from build123d import *

# Parameters (mm, degrees)
BOSS_EXTRUDE1_DEPTH         = 19.05
FILLET1_R                   = 6.35
F_29_0_136_DIAMETER_HOLE1_D = 3.4544


with BuildPart() as part:
    # Sketch1 → Boss-Extrude1 (new body)
    with BuildSketch(Plane.XY):
        with BuildLine():
            ThreePointArc((22.356689849, -6.35), (-23.241, 0), (22.356689849, 6.35))
            Line((22.356689849, 6.35), (57.15, 6.35))
            Line((57.15, 6.35), (57.15, 9.525))
            Line((57.15, 9.525), (24.638981939, 9.525))
            ThreePointArc((24.638981939, 9.525), (-26.416, 0), (24.638981939, -9.525))
            Line((24.638981939, -9.525), (57.15, -9.525))
            Line((57.15, -9.525), (57.15, -6.35))
            Line((57.15, -6.35), (22.356689849, -6.35))
        make_face()
    extrude(amount=BOSS_EXTRUDE1_DEPTH)

    # Fillet1
    fillet1_edges = [part.edges().sort_by_distance(p)[0] for p in [
        (22.356689849, 6.35, 9.525),
        (22.356689849, -6.35, 9.525),
        (24.638981939, -9.525, 9.525),
        (24.638981939, 9.525, 9.525),
    ]]
    fillet(fillet1_edges, radius=FILLET1_R)

    # #29 (0.136) Diameter Hole1 (through all)
    with Locations(Plane(origin=(0, 9.525, 0), x_dir=(1, 0, 0), z_dir=(0, 1, 0))):
        with Locations((33.655, -9.525), (52.705, -9.525)):
            Hole(F_29_0_136_DIAMETER_HOLE1_D / 2)


solid = part.part
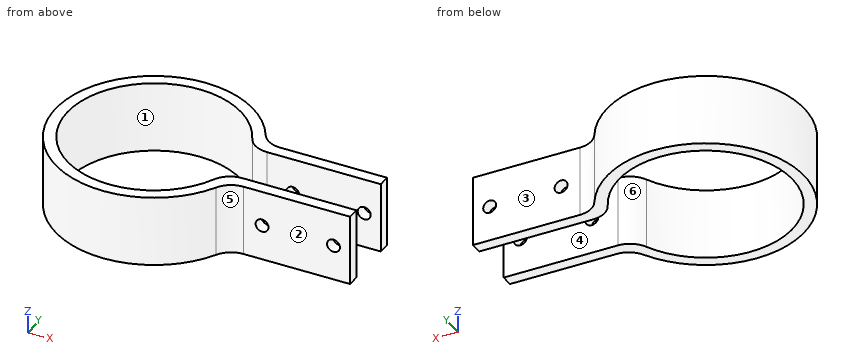
Verification items for the finished model (mm, model axes). Face numbers are marked on the shaded views. A direction names the side the tool comes from. Coordinates: 2 decimals unless noted, no trailing zeros. Loops run counter-clockwise (first coordinate to the right, second up) from the corner with the lowest first, then second, coordinate; pieces in that order, holes last. Notation, with made-up numbers: (-24, 35.5) -> (25, 35.5) arc R29 cw to (25, 62.5) -> close; hole circle Ø11 at (30, -2.75). An arc over 180 degrees is marked (long way). Answer as CSV lines item,"result".
1) Thickness scan on L1, parallel to Y at x = 0, z = 4; L2, parallel to Y at x = 34.5, z = 14.5 (3 decimals); L3, parallel to X at y = -7, z = 5.5. Record the ranges inside material, lowest first. Write a range as from..to.
Found:
L1,"y = -26.42..-23.24, 23.24..26.42"
L2,"y = -9.525..-6.35, 6.35..9.525"
L3,"x = -25.47..-22.16, 23.93..57.15"
2) Cross-section at A-A, the plane x = 0. Record the cut outline in (y, z).
Found:
outline,"(-26.42, 0) -> (-23.24, 0) -> (-23.24, 19.05) -> (-26.42, 19.05) -> close; (23.24, 0) -> (26.42, 0) -> (26.42, 19.05) -> (23.24, 19.05) -> close"
3) Release check for a two-part mould opening along Y. For the marked faces 1, 2 and 3 record: +Y half, -Y half, draft (parallel to the pull), parting line (faces both ways), or undercut.
Found:
face 1,"undercut"
face 2,"-Y half"
face 3,"+Y half"
4) Cross-section at B-B, the plane z = 2.75. Record the cut outline in (x, y) (3 decimals).
Found:
outline,"(20.992, -9.975) arc R23.241 cw (long way) to (20.992, 9.975) arc R6.35 ccw to (26.727, 6.35) -> (57.15, 6.35) -> (57.15, 9.525) -> (28.663, 9.525) arc R6.35 cw to (23.109, 12.798) arc R26.416 ccw (long way) to (23.109, -12.798) arc R6.35 cw to (28.663, -9.525) -> (57.15, -9.525) -> (57.15, -6.35) -> (26.727, -6.35) arc R6.35 ccw to start"
5) Depth check by flat-ended pin: pin 1 (5 mm diameter, centred on x = 18, z = 8, fed in from +Y); pin 2 (8 mm diameter, centred on x = 39, z = 6, fed in from +Y) (3 decimals); pin 3 (6 mm diameter, centred on y = -19.5, z = 13.5, fed in from +X). Enter the tip coordinate at first touch or a pass-through.
Found:
pin 1,"stops at y = 21.39"
pin 2,"stops at y = 9.525"
pin 3,"stops at x = 20.63"
6) Cross-section at D-D, the plane x = 34.5. Record the cut outline in (y, z) (3 decimals), then the cut area to 3 significant figures.
Found:
outline,"(-9.525, 0) -> (-6.35, 0) -> (-6.35, 8.019) -> (-9.525, 8.019) -> close; (-9.525, 11.031) -> (-6.35, 11.031) -> (-6.35, 19.05) -> (-9.525, 19.05) -> close; (6.35, 0) -> (9.525, 0) -> (9.525, 8.019) -> (6.35, 8.019) -> close; (6.35, 11.031) -> (9.525, 11.031) -> (9.525, 19.05) -> (6.35, 19.05) -> close"
area,"102 mm2"
7) Cross-section at C-C, the plane y = -11.5. Record the cut outline in (x, z).
Found:
outline,"(-23.78, 0) -> (-20.2, 0) -> (-20.2, 19.05) -> (-23.78, 19.05) -> close; (20.2, 0) -> (24.06, 0) -> (24.06, 19.05) -> (20.2, 19.05) -> close"
8) Tool access check on the marked faces 4, 5 and 6. Record the directions out of +Z, -Z, +X, -X, +Y, -Y that give a thin tool (end or side, any length) a straight path to the whole face; none if there is none.
Found:
face 4,"+Z, -Z, +X"
face 5,"+Z, -Z, +X, -Y"
face 6,"+Z, -Z"
